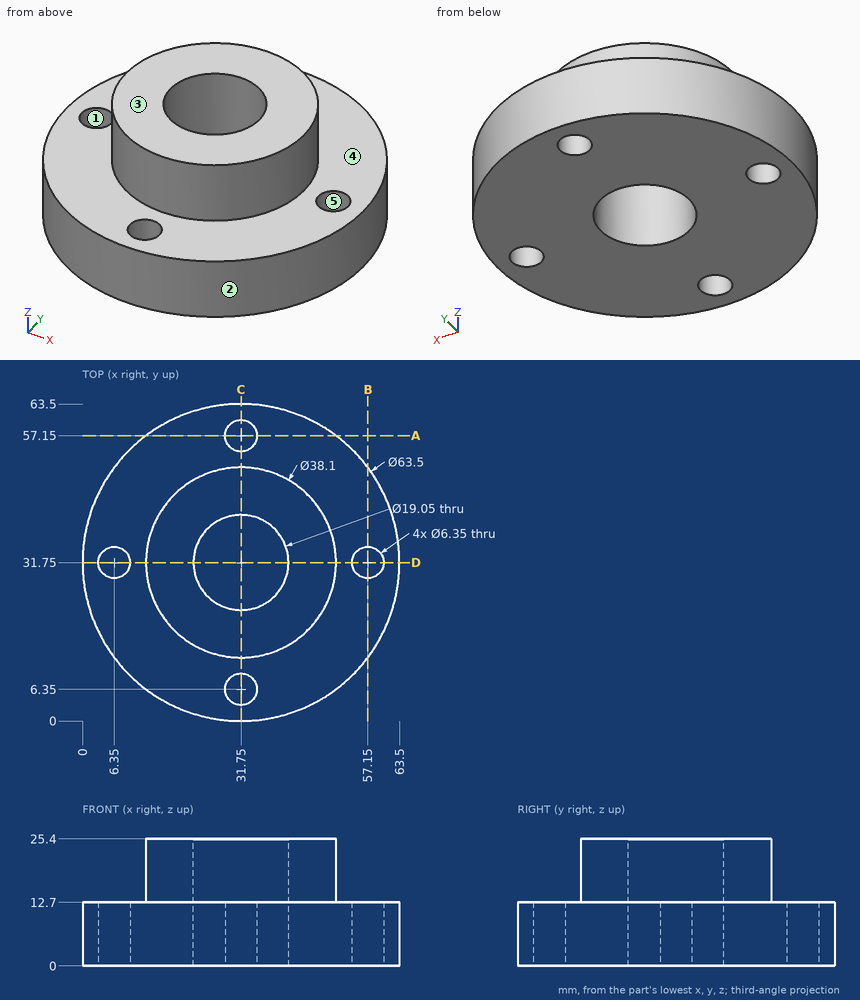
Print and shaded views of the part. All mm, measured from the part's lowest x, y and z. A direction names the side the tool comes from. Coordinates: 2 decimals unless noted, no trailing zeros. Loops run counter-clockwise (first coordinate to the right, second up) from the corner with the lowest first, then second, coordinate; pieces in that order, holes last. Notation, with made-up numbers: (-38, 9) - (-15, 9) arc R26 ccw to (-15, 37) - close; hole circle Ø9 at (23, 37.25). An arc over 180 degrees is marked (long way). Use one line per item in the form item = value. Start each with the question number.
1) Two-plate mould, pull along Y, no slides. Class the marked faces 1, 2 and 3: +Y half, -Y half, draft (parallel to the pull), parting line (faces both ways), or undercut.
2) Tool access for the marked faces 4 and 5: list every direction of +Z, -Z, +X, -X, +Y, -Y with a clear straight run to the whole face (end or side of a thin tool).
3) Band-saw the part on C-C (x = 31.75). Give the cut face in (y, z) (3 decimals).
4) Band-saw the part on A-A (y = 57.15). Give the cut face in (x, z) (3 decimals), and give its area (3 significant figures).
5) Drill centre lines: L1, parallel to Y at x = 31.75, z = 5.5 (3 decimals); L2, parallel to Y at x = 31.75, z = 13.25 (3 decimals); L3, parallel to Y at x = 31, z = 5.25. Where is each one in solid material? Low to high. Write a range as from..to.
6) Flat gauge pins, fed straight in: pin 1 (2 mm diameter, centred on x = 17, z = 6.5, fed in from +Y); pin 2 (4 mm diameter, centred on x = 28, z = 21, fed in from +Y); pin 3 (8 mm diameter, centred on y = 37, z = 21, fed in from +X). Where does each tip first touch, or does it go through?
Check values:
q1.face_1 = undercut
q1.face_2 = parting line
q1.face_3 = draft
q2.face_4 = +Z
q2.face_5 = +Z, -Z
q3.outline = (0, 0) - (3.175, 0) - (3.175, 12.7) - (0, 12.7) - close; (9.525, 0) - (22.225, 0) - (22.225, 25.4) - (12.7, 25.4) - (12.7, 12.7) - (9.525, 12.7) - close; (41.275, 0) - (53.975, 0) - (53.975, 12.7) - (50.8, 12.7) - (50.8, 25.4) - (41.275, 25.4) - close; (60.325, 0) - (63.5, 0) - (63.5, 12.7) - (60.325, 12.7) - close
q4.outline = (12.7, 0) - (28.575, 0) - (28.575, 12.7) - (12.7, 12.7) - close; (34.925, 0) - (50.8, 0) - (50.8, 12.7) - (34.925, 12.7) - close
q4.area = 403 mm2
q5.L1 = 0..3.175, 9.525..22.225, 41.275..53.975, 60.325..63.5
q5.L2 = 12.7..22.225, 41.275..50.8
q5.L3 = 0.01..3.26, 9.44..22.25, 41.25..54.06, 60.24..63.49
q6.pin_1 = 60.37
q6.pin_2 = 50.72
q6.pin_3 = 50.76
